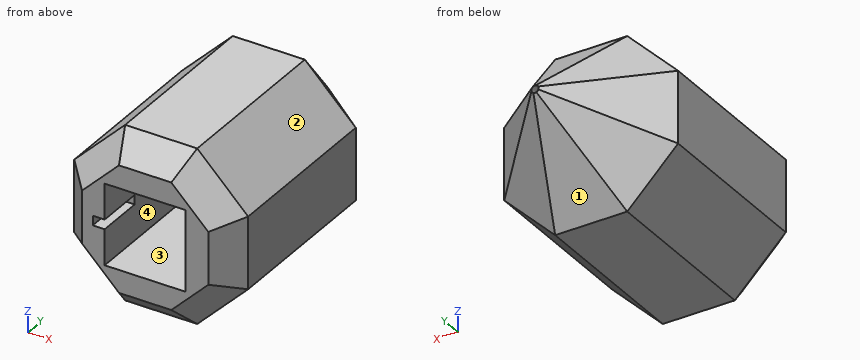
```python
from build123d import *
from OCP.BRepFilletAPI import BRepFilletAPI_MakeChamfer

# Parameters (mm, degrees)
SKETCH1_W           = 34
SKETCH1_H           = 34
BOSS_EXTRUDE1_DEPTH = 120
SKETCH2_W           = 34
SKETCH2_H           = 34
SKETCH2_R           = 1.5
BOSS_EXTRUDE2_DEPTH = 20
SKETCH4_W           = 34
SKETCH4_H           = 34
SKETCH4_R           = 1.5
BOSS_EXTRUDE5_DEPTH = 15
SKETCH3_W           = 34
SKETCH3_H           = 34
SKETCH3_R           = 8
BOSS_EXTRUDE3_DEPTH = 13
CHAMFER1_SIZE       = 37.5
CHAMFER1_SIZE2      = 34.96931573
CHAMFER2_SIZE       = 10
CHAMFER2_SIZE2      = 10.7236871
SKETCH5_W           = 5
SKETCH5_H           = 4
CUT_EXTRUDE1_DEPTH  = 20


with BuildPart() as part:
    # Sketch1 → Boss-Extrude1 (new body)
    with BuildSketch(Plane(origin=(0, 0, 0), x_dir=(1, 0, 0), z_dir=(0, 1, 0))):
        Polygon((-15.136038969, 36.54163056), (-36.54163056, 15.136038969), (-36.54163056, -15.136038969), (-15.136038969, -36.54163056), (15.136038969, -36.54163056), (36.54163056, -15.136038969), (36.54163056, 15.136038969), (15.136038969, 36.54163056), align=None)
        Rectangle(SKETCH1_W, SKETCH1_H, mode=Mode.SUBTRACT)
    extrude(amount=BOSS_EXTRUDE1_DEPTH)

    # Sketch2 → Boss-Extrude2 (add)
    with BuildSketch(Plane(origin=(0, 120, 0), x_dir=(1, 0, 0), z_dir=(0, 1, 0))):
        Polygon((36.54163056, 15.136038969), (15.136038969, 36.54163056), (-15.136038969, 36.54163056), (-36.54163056, 15.136038969), (-36.54163056, -15.136038969), (-15.136038969, -36.54163056), (15.136038969, -36.54163056), (36.54163056, -15.136038969), align=None)
        Rectangle(SKETCH2_W, SKETCH2_H, mode=Mode.SUBTRACT)
        Rectangle(SKETCH2_W, SKETCH2_H)
        with Locations(Location((0, 0, 0), (0, 0, 270))):
            Circle(SKETCH2_R, mode=Mode.SUBTRACT)
    extrude(amount=-BOSS_EXTRUDE2_DEPTH)

    # Sketch4 → Boss-Extrude5 (add)
    with BuildSketch(Plane.XZ.offset(-100)):
        Rectangle(SKETCH4_W, SKETCH4_H)
        with Locations(Location((0, 0, 0), (0, 0, 90))):
            Circle(SKETCH4_R, mode=Mode.SUBTRACT)
    extrude(amount=BOSS_EXTRUDE5_DEPTH)

    # Sketch3 → Boss-Extrude3 (add)
    with BuildSketch(Plane.XZ.offset(-85)):
        Rectangle(SKETCH3_W, SKETCH3_H)
        with Locations(Location((0, 0, 0), (0, 0, 90))):
            Circle(SKETCH3_R, mode=Mode.SUBTRACT)
    extrude(amount=BOSS_EXTRUDE3_DEPTH)

    # Chamfer1: one chamfer whose edges measure the first distance from different faces: ONE call of the kernel's chamfer builder (chamfer() names one face for all edges)
    chamfer1_edges_1 = [part.edges().sort_by_distance(p)[0] for p in [
        (-36.54163056, 120, 0),
    ]]
    chamfer1_side_1 = [part.faces().sort_by_distance(p)[0] for p in [
        (-36.54163056, 60, 0),
    ]]
    chamfer1_edges_2 = [part.edges().sort_by_distance(p)[0] for p in [
        (-25.838834765, 120, 25.838834765),
    ]]
    chamfer1_side_2 = [part.faces().sort_by_distance(p)[0] for p in [
        (-25.838834765, 60, 25.838834765),
    ]]
    chamfer1_edges_3 = [part.edges().sort_by_distance(p)[0] for p in [
        (0, 120, 36.54163056),
    ]]
    chamfer1_side_3 = [part.faces().sort_by_distance(p)[0] for p in [
        (0, 60, 36.54163056),
    ]]
    chamfer1_edges_4 = [part.edges().sort_by_distance(p)[0] for p in [
        (25.838834765, 120, 25.838834765),
    ]]
    chamfer1_side_4 = [part.faces().sort_by_distance(p)[0] for p in [
        (25.838834765, 60, 25.838834765),
    ]]
    chamfer1_edges_5 = [part.edges().sort_by_distance(p)[0] for p in [
        (36.54163056, 120, 0),
    ]]
    chamfer1_side_5 = [part.faces().sort_by_distance(p)[0] for p in [
        (36.54163056, 60, 0),
    ]]
    chamfer1_edges_6 = [part.edges().sort_by_distance(p)[0] for p in [
        (25.838834765, 120, -25.838834765),
    ]]
    chamfer1_side_6 = [part.faces().sort_by_distance(p)[0] for p in [
        (25.838834765, 60, -25.838834765),
    ]]
    chamfer1_edges_7 = [part.edges().sort_by_distance(p)[0] for p in [
        (0, 120, -36.54163056),
    ]]
    chamfer1_side_7 = [part.faces().sort_by_distance(p)[0] for p in [
        (0, 60, -36.54163056),
    ]]
    chamfer1_edges_8 = [part.edges().sort_by_distance(p)[0] for p in [
        (-25.838834765, 120, -25.838834765),
    ]]
    chamfer1_side_8 = [part.faces().sort_by_distance(p)[0] for p in [
        (-25.838834765, 60, -25.838834765),
    ]]
    chamfer1 = BRepFilletAPI_MakeChamfer(part.part.solid().wrapped)
    for e in chamfer1_edges_1:
        chamfer1.Add(CHAMFER1_SIZE, CHAMFER1_SIZE2, e.wrapped, chamfer1_side_1[0].wrapped)  # the first distance lies on this face
    for e in chamfer1_edges_2:
        chamfer1.Add(CHAMFER1_SIZE, CHAMFER1_SIZE2, e.wrapped, chamfer1_side_2[0].wrapped)  # the first distance lies on this face
    for e in chamfer1_edges_3:
        chamfer1.Add(CHAMFER1_SIZE, CHAMFER1_SIZE2, e.wrapped, chamfer1_side_3[0].wrapped)  # the first distance lies on this face
    for e in chamfer1_edges_4:
        chamfer1.Add(CHAMFER1_SIZE, CHAMFER1_SIZE2, e.wrapped, chamfer1_side_4[0].wrapped)  # the first distance lies on this face
    for e in chamfer1_edges_5:
        chamfer1.Add(CHAMFER1_SIZE, CHAMFER1_SIZE2, e.wrapped, chamfer1_side_5[0].wrapped)  # the first distance lies on this face
    for e in chamfer1_edges_6:
        chamfer1.Add(CHAMFER1_SIZE, CHAMFER1_SIZE2, e.wrapped, chamfer1_side_6[0].wrapped)  # the first distance lies on this face
    for e in chamfer1_edges_7:
        chamfer1.Add(CHAMFER1_SIZE, CHAMFER1_SIZE2, e.wrapped, chamfer1_side_7[0].wrapped)  # the first distance lies on this face
    for e in chamfer1_edges_8:
        chamfer1.Add(CHAMFER1_SIZE, CHAMFER1_SIZE2, e.wrapped, chamfer1_side_8[0].wrapped)  # the first distance lies on this face
    add(Compound.cast(chamfer1.Shape()), mode=Mode.REPLACE)

    # Chamfer2
    chamfer2_edges = [part.edges().sort_by_distance(p)[0] for p in [
        (-25.838834765, 0, -25.838834765),
        (0, 0, -36.54163056),
        (25.838834765, 0, -25.838834765),
        (36.54163056, 0, 0),
        (25.838834765, 0, 25.838834765),
        (0, 0, 36.54163056),
        (-25.838834765, 0, 25.838834765),
        (-36.54163056, 0, 0),
    ]]
    chamfer2_side = [part.faces().sort_by_distance(p)[0] for p in [
        (-25.108002154, 0, -25.108002154),
    ]]
    chamfer(chamfer2_edges, length=CHAMFER2_SIZE, length2=CHAMFER2_SIZE2, reference=chamfer2_side[0])

    # Sketch5 → Cut-Extrude1 (cut)
    with BuildSketch(Plane.XZ):
        with Locations((-19.5, 0)):
            Rectangle(SKETCH5_W, SKETCH5_H)
    extrude(amount=-CUT_EXTRUDE1_DEPTH, mode=Mode.SUBTRACT)


solid = part.part
```
Model file for the job. Use its own axes, mm. Face numbers are marked on the shaded views. Coordinates: 2 decimals unless noted, no trailing zeros. Loops run counter-clockwise (first coordinate to the right, second up) from the corner with the lowest first, then second, coordinate; pieces in that order, holes last. Notation, with made-up numbers: (-4.5, -21.5) - (38.5, -21.5) arc R27 cw to (38.5, -4.5) - close; hole circle Ø1 at (57, -22). An arc over 180 degrees is marked (long way). Write item = value, one per line. Start each with the question number.
Item 1: Saw through at A-A, the plane y = 18. List the corners of the cut face in (x, z).
Item 2: Drop flat-ended pins along their axis: pin 1 Ø4 at (x, y) = (-19, 7) entering from +Z; pin 2 Ø17.5 at (x, z) = (0.5, 2.5) entering from -Y; pin 3 Ø5 at (x, z) = (0, 0) entering from -Y. Give the stop position or say it passes through.
Item 3: Saw through at D-D, the plane y = 37. List the corners of the cut face in (x, z).
Item 4: Saw through at B-B, the plane x = -3. List the corners of the cut face in (y, z).
Item 5: Pull direction X, two halves, no side cores. Call the marked faces 1, 2, 3 and 4: +X half, -X half, draft (parallel to the pull), parting line (faces both ways), or undercut.
Item 6: Wall check: probe 1 along X at (y, z) = (52.5, -8.5); probe 2 along X at (y, z) = (91.75, 0). Give the ranges that are in metal, low to high. Write a range as [from, to].
Item 7: Saw through at C-C, the plane z = -19. List the corners of the cut face in (x, y).
Answers:
q1.outline = (-36.54, -15.14) - (-15.14, -36.54) - (15.14, -36.54) - (36.54, -15.14) - (36.54, 15.14) - (15.14, 36.54) - (-15.14, 36.54) - (-36.54, 15.14) - close; hole (-22, -2) - (-17, -2) - (-17, -17) - (17, -17) - (17, 17) - (-17, 17) - (-17, 2) - (-22, 2) - close
q2.pin_1 = 31.08
q2.pin_2 = 72
q2.pin_3 = 85
q3.outline = (-36.54, -15.14) - (-15.14, -36.54) - (15.14, -36.54) - (36.54, -15.14) - (36.54, 15.14) - (15.14, 36.54) - (-15.14, 36.54) - (-36.54, 15.14) - close; hole (-17, -17) - (17, -17) - (17, 17) - (-17, 17) - close
q4.outline = (0, -26.54) - (10.72, -36.54) - (82.5, -36.54) - (113.92, -7.24) - (118.47, -1.24) - (118.47, 1.24) - (113.92, 7.24) - (82.5, 36.54) - (10.72, 36.54) - (0, 26.54) - (0, 17) - (72, 17) - (72, 7.42) - (85, 7.42) - (85, -7.42) - (72, -7.42) - (72, -17) - (0, -17) - close
q5.face_1 = draft
q5.face_2 = +X half
q5.face_3 = undercut
q5.face_4 = undercut
q6.probe_1 = [-36.54, -17], [17, 36.54]
q6.probe_2 = [-27.92, -1.5], [1.5, 27.92]
q7.outline = (-32.68, 10.72) - (-18.54, 0) - (18.54, 0) - (32.68, 10.72) - (32.68, 82.5) - (7.87, 101.31) - (-7.87, 101.31) - (-32.68, 82.5) - close
